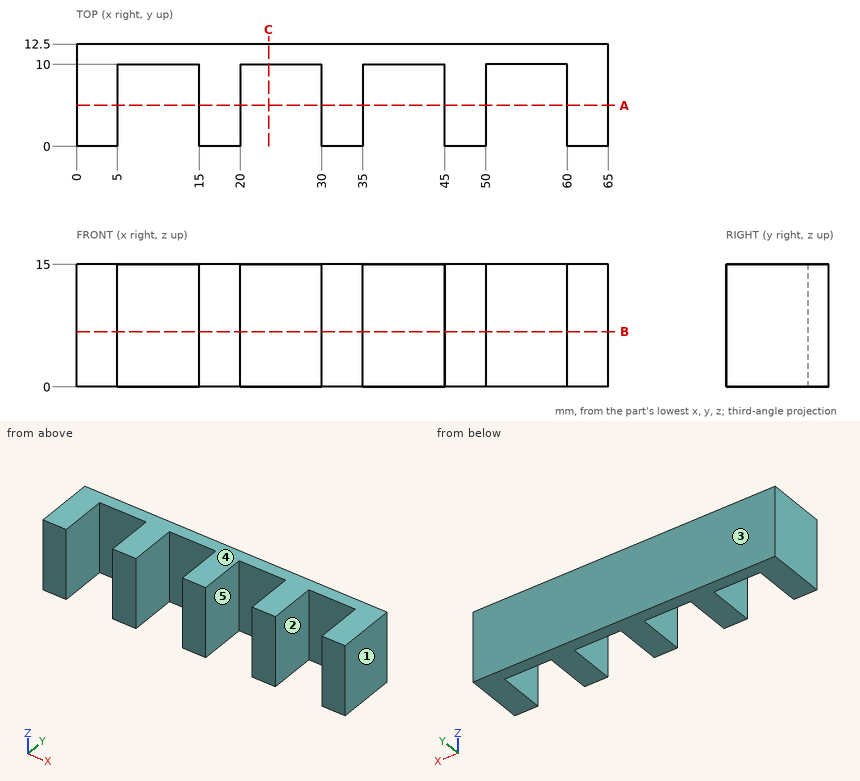
Input: dimensioned drawing with shaded views. Units: mm. Origin: part minimum x, y, z. A direction names the side the tool comes from. Give positions to 0.01 mm unless a question says otherwise; leave off trailing zeros. Order: outer loops, then holes, each group sorted by start corner. A loop starts at its lowest first (then second) coordinate and runs counter-clockwise, first axis right, second up. Notation, with made-up numbers: (52.5, 24.5) -> (91.5, 24.5) arc R11 cw to (91.5, 43.5) -> close; hole circle Ø4 at (19, 49). An arc over 180 degrees is marked (long way). Use one line per item in the form item = value.
1) Section C-C, the plane x = 23.5. Return loops of the section in (y, z).
Response values:
outline = (10, 0) -> (12.5, 0) -> (12.5, 15) -> (10, 15) -> close
2) Section B-B, the plane z = 6.75. Return loops of the section in (x, y).
Response values:
outline = (0, 0) -> (5, 0) -> (5, 10) -> (15, 10) -> (15, 0) -> (20, 0) -> (20, 10) -> (30, 10) -> (30, 0) -> (35, 0) -> (35, 10) -> (45, 10) -> (45, 0) -> (50, 0) -> (50, 10) -> (60, 10) -> (60, 0) -> (65, 0) -> (65, 12.5) -> (0, 12.5) -> close
3) First-contact query: pin 1 Ø5 at (x, z) = (24.5, 7.5) entering from -Y. Flat tip, straight axial feed; report the tip coordinate or a pass-through.
Response values:
pin_1 = 10
4) Reachability of the marked faces 4 and 5 from +Z, -Z, +X, -X, +Y, -Y: full face, straight path, thin tool, end or side. Return the list, or none.
Response values:
face_4 = +Z, +X, -X, +Y, -Y
face_5 = +Z, -Z, -Y
5) Section A-A, the plane y = 5. Return loops of the section in (x, z).
Response values:
outline = (0, 0) -> (5, 0) -> (5, 15) -> (0, 15) -> close; (15, 0) -> (20, 0) -> (20, 15) -> (15, 15) -> close; (30, 0) -> (35, 0) -> (35, 15) -> (30, 15) -> close; (45, 0) -> (50, 0) -> (50, 15) -> (45, 15) -> close; (60, 0) -> (65, 0) -> (65, 15) -> (60, 15) -> close
6) Line query: probe 1 along X at (y, z) = (9.75, 10.5); probe 2 along Y at (x, z) = (35.5, 10). Output: solid intervals per line, ascending.
Response values:
probe_1 = 0 to 5, 15 to 20, 30 to 35, 45 to 50, 60 to 65
probe_2 = 10 to 12.5
7) Mould query, pull axis X, two halves, no side actions, for the marked faces 1, 2 and 3. Classes: pulls with the +X half, pulls with the -X half, needs draft (parallel to the pull), parting line crosses it, or undercut.
Response values:
face_1 = pulls with the +X half
face_2 = undercut
face_3 = needs draft
